```python
from build123d import *

# Parameters (mm, degrees)
SKETCH_8_R               = 2.25
EXTRUDE_23_DEPTH         = 6.3
EXTRUDE_24_DEPTH         = 3.8
SKETCH_8_5_R             = 1
CUT_EXTRUDE_2_DEPTH      = 37.420049423
PATTERN_CIRCULAR_1_COUNT = 3
CUT_EXTRUDE_3_DEPTH      = 3.7
PATTERN_CIRCULAR_2_COUNT = 3
CUT_EXTRUDE_6_DEPTH      = 1
SKETCH_12_W              = 12
SKETCH_12_H              = 8
SKETCH_12_W_2            = 11
SKETCH_12_H_2            = 7
EXTRUDE_1_DEPTH          = 4
SKETCH_14_R              = 6.2
SKETCH_14_R_2            = 4.5
CUT_EXTRUDE_7_DEPTH      = 1
FILLET_1_R               = 0.5
EXTRUDE_25_DEPTH         = 2.5
EXTRUDE_26_OUTLINE_R     = 1.7
EXTRUDE_26_DEPTH         = 2


# Read off the part's stored shape, not the designer's step: 凸台-拉伸26
with BuildPart() as part:
    # 草图7 → 旋转1 (revolve)
    with BuildSketch(Plane.XY, mode=Mode.PRIVATE) as revolve_1_sk:
        Polygon((0, 0), (24.6, 0), (25.3, 7.8), (24.8, 7.8), (24.755128205, 7.3), (24.255128205, 7.3), (23.68974359, 1), (0, 1), align=None)
    revolve(revolve_1_sk.sketch.rotate(Axis((0, 1, 0), (0, -1, 0)), 180), axis=Axis((0, 1, 0), (0, -1, 0)))

    # 草图8 → 凸台-拉伸23 (add)
    with BuildSketch(Plane(origin=(0, 1, 0), x_dir=(1, 0, 0), z_dir=(0, 1, 0))):
        with Locations((0, 22.05)):
            Circle(SKETCH_8_R)
    extrude_23 = extrude(amount=EXTRUDE_23_DEPTH)

    # 草图8<4> → 凸台-拉伸24 (add)
    with BuildSketch(Plane(origin=(0, 1, 0), x_dir=(1, 0, 0), z_dir=(0, 1, 0))):
        with BuildLine():
            Line((-3, 22.05), (-3, 24.114103757))
            ThreePointArc((-3, 24.114103757), (0, 24.3), (3, 24.114103757))
            Line((3, 24.114103757), (3, 22.05))
            ThreePointArc((3, 22.05), (0, 19.05), (-3, 22.05))
        make_face()
    extrude_24 = extrude(amount=EXTRUDE_24_DEPTH)

    # 草图8<5> → 切除-拉伸2 (cut, symmetric)
    with BuildSketch(Plane(origin=(0, 1, 0), x_dir=(1, 0, 0), z_dir=(0, 1, 0))):
        with Locations(Location((0, 22.05, 0), (0, 0, 180))):
            Circle(SKETCH_8_5_R)
    cut_extrude_2 = extrude(amount=CUT_EXTRUDE_2_DEPTH, both=True, mode=Mode.SUBTRACT)

    # 阵列(圆周)1: 凸台-拉伸23, 凸台-拉伸24, 切除-拉伸2 ×3 about axis
    pattern_circular_1_axis = Axis((0, 0, 0), (0, 1, 0))
    add([extrude_23.rotate(pattern_circular_1_axis, i * 360 / PATTERN_CIRCULAR_1_COUNT) for i in range(1, PATTERN_CIRCULAR_1_COUNT)])
    add([extrude_24.rotate(pattern_circular_1_axis, i * 360 / PATTERN_CIRCULAR_1_COUNT) for i in range(1, PATTERN_CIRCULAR_1_COUNT)])
    add([cut_extrude_2.rotate(pattern_circular_1_axis, i * 360 / PATTERN_CIRCULAR_1_COUNT) for i in range(1, PATTERN_CIRCULAR_1_COUNT)], mode=Mode.SUBTRACT)

    # 草图9 → 切除-拉伸3 (cut)
    with BuildSketch(Plane.XZ):
        with BuildLine():
            Line((2, -22.05), (2, -26.095171051))
            Line((2, -26.095171051), (-2, -26.095171051))
            Line((-2, -26.095171051), (-2, -22.05))
            ThreePointArc((-2, -22.05), (0, -20.05), (2, -22.05))
        make_face()
    cut_extrude_3 = extrude(amount=-CUT_EXTRUDE_3_DEPTH, mode=Mode.SUBTRACT)

    # 阵列(圆周)2: 切除-拉伸3 ×3 about axis
    pattern_circular_2_axis = Axis((0, 0, 0), (0, 1, 0))
    for i in range(1, PATTERN_CIRCULAR_2_COUNT):
        add(cut_extrude_3.rotate(pattern_circular_2_axis, i * 360 / PATTERN_CIRCULAR_2_COUNT), mode=Mode.SUBTRACT)

    # 草图11 → 切除-拉伸6 (cut)
    with BuildSketch(Plane(origin=(0, 1, 0), x_dir=(1, 0, 0), z_dir=(0, 1, 0))):
        Polygon((10.3, 15.375), (10.3, 4.675), (17, 4.675), (19, 6.675), (19, 13.375), (17, 15.375), align=None)
        Polygon((14.3, 3.675), (14.3, -7.025), (21, -7.025), (23, -5.025), (23, 1.675), (21, 3.675), align=None)
    extrude(amount=-CUT_EXTRUDE_6_DEPTH, mode=Mode.SUBTRACT)

    # 草图12 → 拉伸-薄壁1 (add)
    with BuildSketch(Plane(origin=(0, 1, 0), x_dir=(1, 0, 0), z_dir=(0, 1, 0))):
        with Locations((0, -16.8)):
            Rectangle(SKETCH_12_W, SKETCH_12_H)
        with Locations((0, -16.8)):
            Rectangle(SKETCH_12_W_2, SKETCH_12_H_2, mode=Mode.SUBTRACT)
    extrude(amount=EXTRUDE_1_DEPTH)

    # 草图14 → 切除-拉伸7 (cut)
    with BuildSketch(Plane(origin=(0, 1, 0), x_dir=(1, 0, 0), z_dir=(0, 1, 0))):
        with Locations(Location((0, 0, 0), (0, 0, 180))):
            Circle(SKETCH_14_R)
        with Locations(Location((11.70765428, -15.20450888, 0), (0, 0, 180))):
            Circle(SKETCH_14_R_2)
    extrude(amount=-CUT_EXTRUDE_7_DEPTH, mode=Mode.SUBTRACT)

    # 圆角1
    fillet_1_edges = [part.edges().sort_by_distance(p)[0] for p in [
        (17.363809346, 0, 10.025),
        (21.164779892, 0, 9.910090291),
        (-21.164779892, 0, 9.910090291),
        (-17.363809346, 0, 10.025),
        (-19.164779892, 0, 13.374191906),
        (-18.088117647, 0, -16.67273223),
        (-2, 0, -23.284282198),
        (0, 0, -20.05),
        (2, 0, -23.284282198),
        (21.304224933, 0, -12.3),
        (19.164779892, 0, 13.374191906),
        (0, 0, 24.6),
    ]]
    fillet(fillet_1_edges, radius=FILLET_1_R)

    # 草图15 → 凸台-拉伸25 (add)
    with BuildSketch(Plane(origin=(0, 1, 0), x_dir=(1, 0, 0), z_dir=(0, 1, 0))):
        Polygon((0.75, -17.55), (5.5, -17.55), (5.5, -16.05), (0.75, -16.05), (0.75, -13.3), (-0.75, -13.3), (-0.75, -16.05), (-5.5, -16.05), (-5.5, -17.55), (-0.75, -17.55), (-0.75, -20.3), (0.75, -20.3), align=None)
    extrude(amount=EXTRUDE_25_DEPTH)

    # 凸台-拉伸26 outline → 凸台-拉伸26 (add)
    with BuildSketch(Plane(origin=(0, 1, 0), x_dir=(1, 0, 0), z_dir=(0, 1, 0))):
        with BuildLine():
            Line((11.322847478, 4.675), (10.807173544, 4.675))
            ThreePointArc((10.807173544, 4.675), (-10.566173989, -5.196786722), (10.3, 5.706191812))
            Line((10.3, 5.706191812), (10.3, 6.631176366))
            ThreePointArc((10.3, 6.631176366), (-10.855576433, -5.676174795), (11.322847478, 4.675))
        make_face()
        with Locations((0, 9)):
            Circle(EXTRUDE_26_OUTLINE_R)
        with Locations((7.794228634, -4.5)):
            Circle(EXTRUDE_26_OUTLINE_R)
        with Locations((-7.794228634, -4.5)):
            Circle(EXTRUDE_26_OUTLINE_R)
    extrude(amount=EXTRUDE_26_DEPTH)


solid = part.part
```
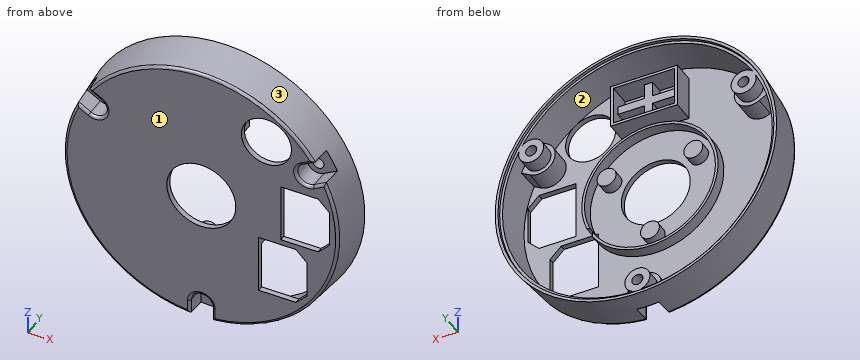
CAD build for the part. Positions are in the model's coordinates, mm. Face numbers are marked on the shaded views. Round coordinates to 2 decimals unless told otherwise and drop trailing zeros. Return JSON: item names as keys, results as strings. Group by question number.
(1) Mould opens along X. For the marked faces 1, 2 and 3 say: +X half, -X half, draft (parallel to the pull), parting line (faces both ways), or undercut.
(2) Wall check: probe 1 along X at (y, z) = (2, -2.5); probe 2 along Z at (x, y) = (19, 5.75); probe 3 along Z at (x, y) = (-0.5, 2.25). Give the ranges that are in metal, low to high. Write a range as [from, to].
(3) Saw through at A-A, the plane z = 0. Give the number of separate pieces and of enclosed holes in the cut face, and give its area (3 significant figures).
(4) Drop flat-ended pins along their axis: P1, Ø2.5, axis at x = 1, z = -22, coming from the +Y side; P2, Ø4.5, axis at x = 2.5, y = 3, coming from the +Z side; P3, Ø2.5, axis at x = 0, z = -22.05, coming from the -Y side. Give the stop position or say it passes through.
Answer list:
{
 "1": {"face 1": "draft", "face 2": "undercut", "face 3": "parting line"},
 "2": {"probe 1": "[-24.65, -23.65], [-11.99, -11.51], [11.51, 11.99], [23.65, 24.65]", "probe 2": "[-16.43, -14.85], [8.78, 10.03], [12.02, 13.27], [14.85, 16.43]", "probe 3": "[-20.11, -19.09], [-12.24, -11.76], [-10.62, -7.38], [11.76, 12.24], [12.8, 20.8], [23.8, 24.8]"},
 "3": {"separate pieces": "3", "enclosed holes": "0", "area": "43.1 mm2"},
 "4": {"P1": "y = 7.3", "P2": "z = 25.01", "P3": "y = 3.7"}
}
